Design review of the part built by this model. Coordinates are the model's own, in mm. Face numbers are marked on the shaded views. Coordinates: 2 decimals unless noted, no trailing zeros. Loops run counter-clockwise (first coordinate to the right, second up) from the corner with the lowest first, then second, coordinate; pieces in that order, holes last. Notation, with made-up numbers: (38, 67.25) -> (69, 67.25) arc R25 cw to (69, 105.25) -> close; hole circle Ø9 at (13, -4.75). An arc over 180 degrees is marked (long way). Answer as a JSON object with one key per item and string values.
```python
from build123d import *

# Parameters (mm, degrees)
F0_W     = 76.2
F0_H     = 76.2
F1_DEPTH = 170.942
F2_R     = 25.000448
F3_DEPTH = 76.201
F4_R     = 50.8


with BuildPart() as f1:
    # F0 (on Front) → F1 (new body)
    with BuildSketch(Plane.XZ):
        Rectangle(F0_W, F0_H)
    extrude(amount=F1_DEPTH)

    # F2 (on face) → F3 (cut, through all)
    with BuildSketch(Plane.XY.offset(38.1)):
        with Locations((0, -126.970813)):
            Circle(F2_R)
    extrude(amount=-F3_DEPTH, mode=Mode.SUBTRACT)

    # F4
    f4_edges = [f1.edges().sort_by_distance(p)[0] for p in [
        (38.1, -170.942, 0),
    ]]
    fillet(f4_edges, radius=F4_R)


solid = f1.part
```
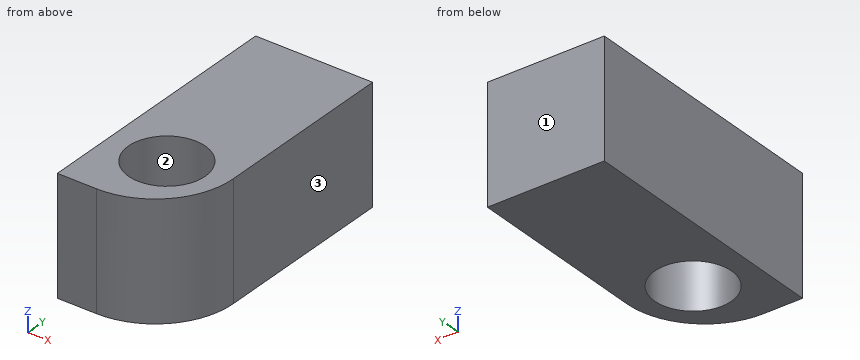
1) Add section C-C, the plane z = 32.5. Give the boundary of the cut face in (x, y).
Completed:
{"outline": "(-38.1, -170.94) -> (-12.7, -170.94) arc R50.8 ccw to (38.1, -120.14) -> (38.1, 0) -> (-38.1, 0) -> close; hole circle Ø50 at (0, -126.97)"}
2) Clearance check with flat-ended pins moving along their axes: pin 1 Ø12 at (x, z) = (-7, -13) entering from -Y; pin 2 Ø12 at (x, z) = (-3.5, -10) entering from -Y; pin 3 Ø4 at (x, z) = (9, 6) entering from -Y. State where each tip first meets the part, or that it passes through.
Completed:
{"pin 1": "y = -170.94", "pin 2": "y = -170.84", "pin 3": "y = -166.97"}
3) Wall thickness on probe 1 along Y at (x, z) = (2, -28); probe 2 along X at (y, z) = (-116, -8.5); probe 3 along Y at (x, z) = (0, -8): over which ranges is each line inside the solid? List them lowest first.
Completed:
{"probe 1": "-168.77 to -151.89, -102.05 to 0", "probe 2": "-38.1 to -22.46, 22.46 to 38.1", "probe 3": "-169.33 to -151.97, -101.97 to 0"}
4) Add section A-A, the plane y = -139. Give the boundary of the cut face in (x, z).
Completed:
{"outline": "(-38.1, -38.1) -> (-21.92, -38.1) -> (-21.92, 38.1) -> (-38.1, 38.1) -> close; (21.92, -38.1) -> (34.47, -38.1) -> (34.47, 38.1) -> (21.92, 38.1) -> close"}
5) The part is to be moulded in two halves that separate along X. For the marked faces 1, 2 and 3, say which applies: pulls with the +X half, pulls with the -X half, needs draft (parallel to the pull), parting line crosses it, or undercut.
Completed:
{"face 1": "needs draft", "face 2": "undercut", "face 3": "pulls with the +X half"}
6) Add section B-B, the plane x = -22. Give the boundary of the cut face in (y, z), and give its area (3 significant figures).
Completed:
{"outline": "(-170.94, -38.1) -> (-138.85, -38.1) -> (-138.85, 38.1) -> (-170.94, 38.1) -> close; (-115.1, -38.1) -> (0, -38.1) -> (0, 38.1) -> (-115.1, 38.1) -> close", "area": "11,200 mm²"}
